from build123d import *

# Parameters (mm, degrees)
SKETCH1_R           = 45
SKETCH1_R_2         = 5
BOSS_EXTRUDE1_DEPTH = 2.5
BOSS_EXTRUDE2_DEPTH = 10
CIRPATTERN3_COUNT   = 9
BOSS_EXTRUDE6_DEPTH = 10
CIRPATTERN4_COUNT   = 9


with BuildPart() as part:
    # Sketch1 → Boss-Extrude1 (new body)
    with BuildSketch(Plane.XY):
        Circle(SKETCH1_R)
        Circle(SKETCH1_R_2, mode=Mode.SUBTRACT)
    boss_extrude1 = extrude(amount=BOSS_EXTRUDE1_DEPTH)

    # Sketch2 → Boss-Extrude2 (add)
    with BuildSketch(Plane(origin=(0, 0, 0), x_dir=(-1, 0, 0), z_dir=(0, 0, -1))):
        with BuildLine():
            Line((2.376945651, 27.919273565), (2.996801322, 28.703989404))
            ThreePointArc((2.996801322, 28.703989404), (-1.593989447, 32.774038165), (-5.693957299, 37.338128482))
            ThreePointArc((-5.693957299, 37.338128482), (-1.825718804, 40.535941838), (0.472898867, 44.997515117))
            ThreePointArc((0.472898867, 44.997515117), (-0.028187178, 44.999991172), (-0.529269728, 44.996887376))
            ThreePointArc((-0.529269728, 44.996887376), (-2.71555077, 40.967370456), (-6.298348731, 38.107232317))
            ThreePointArc((-6.298348731, 38.107232317), (-8.321118794, 40.910790025), (-10.160523263, 43.837926126))
            ThreePointArc((-10.160523263, 43.837926126), (-10.667701719, 43.717275076), (-11.173448403, 43.590756483))
            ThreePointArc((-11.173448403, 43.590756483), (-5.142118978, 35.111827702), (2.376945651, 27.919273565))
        make_face()
    boss_extrude2 = extrude(amount=BOSS_EXTRUDE2_DEPTH)

    # CirPattern3: Boss-Extrude2 ×9 about axis
    cirpattern3_axis = Axis((0, 0, 0), (0, 0, 1))
    for i in range(1, CIRPATTERN3_COUNT):
        add(boss_extrude2.rotate(cirpattern3_axis, i * 360 / CIRPATTERN3_COUNT))

    # Sketch3 → Boss-Extrude6 (add)
    with BuildSketch(Plane(origin=(0, 0, 0), x_dir=(-1, 0, 0), z_dir=(0, 0, -1))):
        with BuildLine():
            ThreePointArc((0.145366303, 43.995082638), (9.96868345, 42.851065074), (19.288277599, 39.541759887))
            ThreePointArc((19.288277599, 39.541759887), (19.371803139, 40.058594285), (19.460240105, 40.574610966))
            ThreePointArc((19.460240105, 40.574610966), (10.208967999, 43.826669648), (0.472898867, 44.997515117))
            ThreePointArc((0.472898867, 44.997515117), (0.31970879, 44.492843232), (0.145366303, 43.995082638))
        make_face()
    boss_extrude6 = extrude(amount=BOSS_EXTRUDE6_DEPTH)

    # CirPattern4: Boss-Extrude6 ×9 about axis
    cirpattern4_axis = Axis((0, 0, 2.5), (0, 0, -1))
    for i in range(1, CIRPATTERN4_COUNT):
        add(boss_extrude6.rotate(cirpattern4_axis, i * 360 / CIRPATTERN4_COUNT))

    # Mirror3: Boss-Extrude1 across plane
    add(boss_extrude1.mirror(Plane.XY.offset(-5)))


solid = part.part
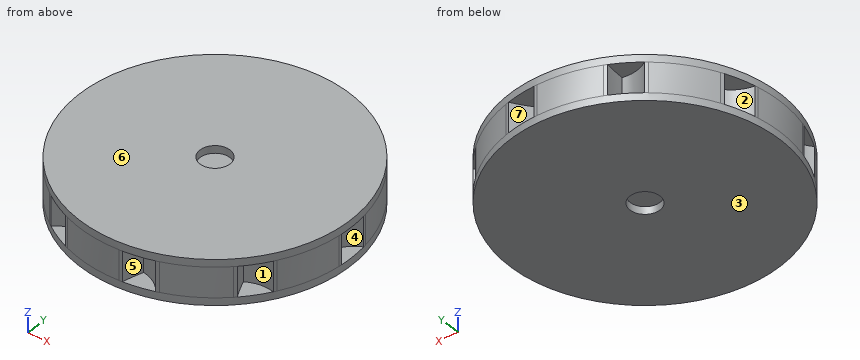
The model under review builds one solid part; all positions refer to its coordinate system, in mm. Face numbers are marked on the shaded views. A direction names the side the tool comes from. Give positions to 0.01 mm unless a question says otherwise; leave off trailing zeros. Order: outer loops, then holes, each group sorted by start corner. A loop starts at its lowest first (then second) coordinate and runs counter-clockwise, first axis right, second up. Notation, with made-up numbers: M 38.25,16 L 53.25,16 A23 cw 53.25,30 Z; hole C 8,35.25 d11. An arc over 180 degrees is marked long. Use one line per item in the form item = value. Start each with the question number.
Item 1: The part is to be moulded in two halves that separate along X. For the marked faces 1, 2, 3 and 4, say which applies: pulls with the +X half, pulls with the -X half, needs draft (parallel to the pull), parting line crosses it, or undercut.
Item 2: We need section A-A on x = 3. Give the boundary of the cut face in (y, z), plus the area to 3 significant figures.
Item 3: Insertion check: pin 1 Ø9 at (x, y) = (0, 0) entering from +Z; pin 2 Ø5 at (x, z) = (-15, -10.5) entering from -Y; pin 3 Ø4 at (y, z) = (19, -7) entering from -X; pin 4 Ø4 at (x, z) = (-26.5, -9) entering from -Y. Each pin has a flat end and moves straight along its axis. Give the tip position at first contact, or say it passes through.
Item 4: To check wall thickness, follow line 1 along Z through (x, y) = (-8, -30); line 2 along Y through (x, z) = (0, 0.6); line 3 along X through (y, z) = (-32, -3.25). State the ranges of each line that lie inside material, in increasing order. Write a range as from..to.
Item 5: For the marked faces 5, 6 and 7, list the 3-axis set-ups (+Z, -Z, +X, -X, +Y, -Y) from which the entire face can be reached by the end or side of a thin tool; tool diameter is ignored.
Item 6: We need section B-B on x = 34. Give the boundary of the cut face in (y, z), plus the area to 3 significant figures.
Completed:
q1.face_1 = undercut
q1.face_2 = pulls with the -X half
q1.face_3 = needs draft
q1.face_4 = pulls with the +X half
q2.outline = M -44.9,-12.5 L -4,-12.5 L -4,-10 L -43.89,-10 L -43.89,0 L -4,0 L -4,2.5 L -44.9,2.5 Z; M 4,-12.5 L 44.9,-12.5 L 44.9,-10 L 40.64,-10 L 40.64,0 L 44.9,0 L 44.9,2.5 L 4,2.5 L 4,0 L 32.77,0 L 32.77,-10 L 4,-10 Z; hole M 34.22,-10 L 39.27,-10 L 39.27,0 L 34.22,0 Z
q2.area = 447 mm²
q3.pin_1 = through
q3.pin_2 = -43.23
q3.pin_3 = -41.41
q3.pin_4 = -37.72
q4.line_1 = -12.5..-10, 0..2.5
q4.line_2 = -45..-5, 5..45
q4.line_3 = -31.64..-30.19, -18.17..-16.16, 8.31..9.41, 30.19..31.64
q5.face_5 = -Y
q5.face_6 = +Z, +X, -X, +Y, -Y
q5.face_7 = +Y
q6.outline = M -29.48,-12.5 L 29.48,-12.5 L 29.48,-10 L 26.39,-10 L 26.39,0 L 29.48,0 L 29.48,2.5 L -29.48,2.5 L -29.48,0 L -22.86,0 L -22.86,-10 L -29.48,-10 Z; hole M -21.88,-10 L 1.94,-10 L 1.94,0 L -21.88,0 Z; hole M 3.14,-10 L 25.34,-10 L 25.34,0 L 3.14,0 Z
q6.area = 327 mm²
